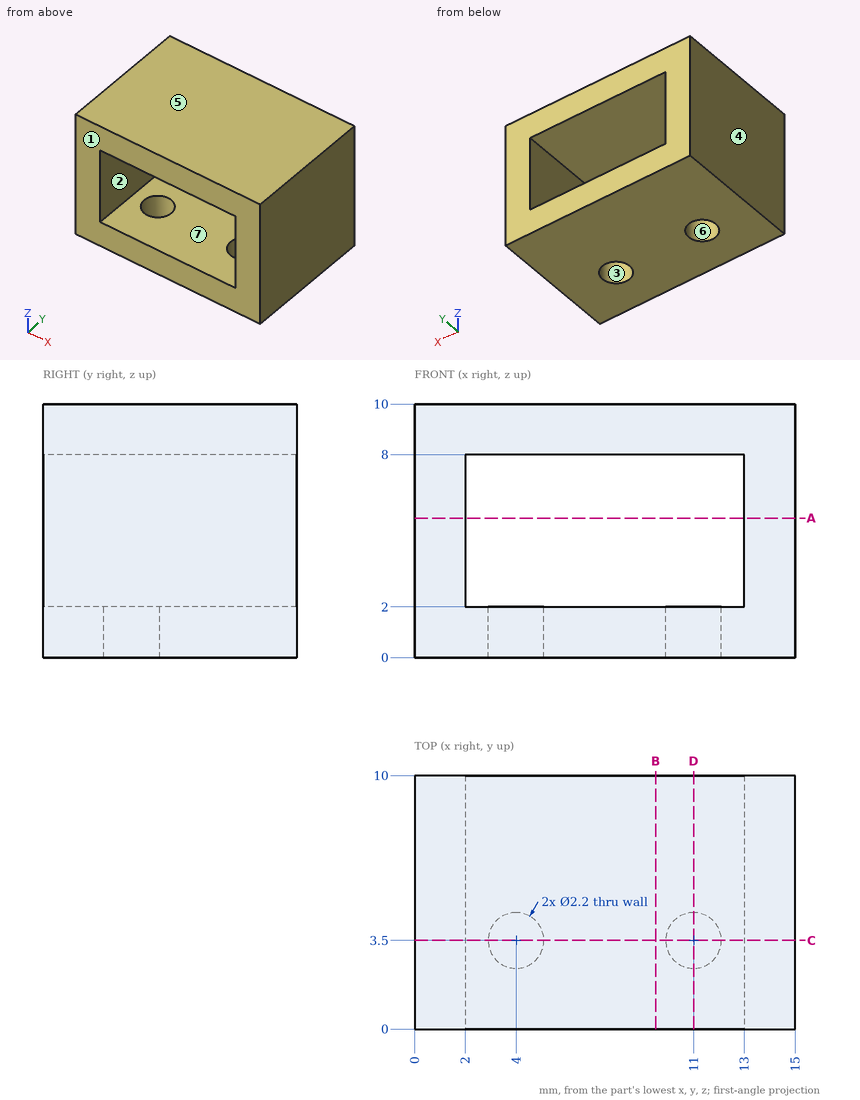
Geometry: see drawing. Coordinates: mm, zero at the bounding-box minimum. A direction names the side the tool comes from. Round coordinates to 2 decimals unless told otherwise and drop trailing zeros. Order: outer loops, then holes, each group sorted by start corner. A loop starts at its lowest first (then second) coordinate and runs counter-clockwise, first axis right, second up. Notation, with made-up numbers: (12.5, 45.25) - (52.5, 45.25) arc R10 cw to (52.5, 59.25) - close; hole circle Ø2 at (35, -3.5). An arc over 180 degrees is marked (long way). Use a Markdown table: item, result. Add a question column.
1. Line query: probe 1 along X at (y, z) = (3.5, 1.35); probe 2 along X at (y, z) = (8.25, 3.25); probe 3 along Z at (x, y) = (11.75, 4.5). Output: solid intervals per line, ascending.
2. Section query B-B (x = 9.5). Return the cut outline in (y, z).
3. Section query D-D (x = 11). Return the cut outline in (y, z), then the cut area to 3 significant figures.
4. Set-up query: the marked faces 1, 2 and 3. Return all of +Z, -Z, +X, -X, +Y, -Y with unobstructed straight access to the full face (end or side cutting, diameter ignored); none if empty.
5. Section query A-A (z = 5.5). Return the cut outline in (x, y), then the cut area to 3 significant figures.
6. Mould query, pull axis X, two halves, no side actions, for the marked faces 4, 5, 6 and 7. Classes: +X half, -X half, draft (parallel to the pull), parting line (faces both ways), or undercut.
7. Section query C-C (y = 3.5). Return the cut outline in (x, z).
Derived:
| question | item | result |
|---|---|---|
| 1 | probe 1 | 0 to 2.9, 5.1 to 9.9, 12.1 to 15 |
| 1 | probe 2 | 0 to 2, 13 to 15 |
| 1 | probe 3 | 0 to 2, 8 to 10 |
| 2 | outline | (0, 0) - (10, 0) - (10, 2) - (0, 2) - close; (0, 8) - (10, 8) - (10, 10) - (0, 10) - close |
| 3 | outline | (0, 0) - (2.4, 0) - (2.4, 2) - (0, 2) - close; (0, 8) - (10, 8) - (10, 10) - (0, 10) - close; (4.6, 0) - (10, 0) - (10, 2) - (4.6, 2) - close |
| 3 | area | 35.6 mm2 |
| 4 | face 1 | +Z, -Z, +X, -X, -Y |
| 4 | face 2 | +Y, -Y |
| 4 | face 3 | -Z |
| 5 | outline | (0, 0) - (2, 0) - (2, 10) - (0, 10) - close; (13, 0) - (15, 0) - (15, 10) - (13, 10) - close |
| 5 | area | 40.0 mm2 |
| 6 | face 4 | -X half |
| 6 | face 5 | draft |
| 6 | face 6 | undercut |
| 6 | face 7 | undercut |
| 7 | outline | (0, 0) - (2.9, 0) - (2.9, 2) - (2, 2) - (2, 8) - (13, 8) - (13, 2) - (12.1, 2) - (12.1, 0) - (15, 0) - (15, 10) - (0, 10) - close; (5.1, 0) - (9.9, 0) - (9.9, 2) - (5.1, 2) - close |
